The listing builds one solid part. Answer for the finished solid, in the listing's coordinates (mm). A direction names the side the tool comes from. Coordinates: 2 decimals unless noted, no trailing zeros. Loops run counter-clockwise (first coordinate to the right, second up) from the corner with the lowest first, then second, coordinate; pieces in that order, holes last. Notation, with made-up numbers: M 27.5,43.5 L 52.5,43.5 A33 ccw 52.5,78.5 Z; hole C 3.5,19 d9. An arc over 180 degrees is marked long. Return JSON: item names as keys, results as strings. Group by question number.
1. Given P1, Ø1.9, axis at x = -28.375, z = -12, coming from the -Y side; P2, Ø3.5, axis at x = 0, z = 11, coming from the -Y side (3 decimals); P3, Ø6.5, axis at x = 0, z = 19, coming from the +Y side, each flat-ended and moving along its own axis, determine where each tip first touches the part or whether it passes through.
2. Which of the six approach directions +Z, -Z, +X, -X, +Y, -Y give full straight-line access (tool end or side, diameter ignored) to faces 5 (the face through (-2.72, 5.118, 15.453)), 6 (the face through (12.69, 1.61, -12.59)), 7 (the face through (9.487, 4.74, -0.336))?
3. Section D-D (y = 2) is taken. Count the separate pieces of the cut face and the enclosed holes in it, then the cut area to 3 significant figures.
4. The mould has two halves that part along X. Classify faces 1 (the face through (-15.35, 3.13, 20.23)), 2 (the face through (-40, 3, 0)), 3 (the face through (18, 3.85, 2)), 4 (the face through (8, 6.35, -6)): pulls with the +X half, pulls with the -X half, needs draft (parallel to the pull), parting line crosses it, or undercut.
5. Section B-B (z = 20) is taken. Write down the section's boundary in (x, y) (3 decimals).
6. Straight lines are drawn through the part: L1, parallel to X at y = 2.25, z = 20 (3 decimals); L2, parallel to Z at x = -11, y = 5.3; L3, parallel to X at y = 0.75, z = -1.5. For each, find the intervals that lie inside material, in ascending order. Write a range as from..to.
7. Section C-C (z = -3) is taken. Write down the section's boundary in (x, y) (3 decimals).
8. Section A-A (x = 19) is taken. Write down the section's boundary in (y, z).
```python
from build123d import *

# Parameters (mm, degrees)
SKETCH1_W           = 80
SKETCH1_H           = 55
SKETCH1_R           = 1.55
SKETCH1_R_2         = 2.05
SKETCH1_R_3         = 1.05
SKETCH1_R_4         = 1.35
SKETCH1_R_5         = 9
BOSS_EXTRUDE1_DEPTH = 6.35
SKETCH3_R           = 4.47
CUT_EXTRUDE2_DEPTH  = 2.5
SKETCH2_W           = 29
SKETCH2_H           = 29
CUT_EXTRUDE1_DEPTH  = 3.175
FILLET1_R           = 6.35


with BuildPart() as part:
    # Sketch1 → Boss-Extrude1 (new body)
    with BuildSketch(Plane(origin=(0, 0, 0), x_dir=(1, 0, 0), z_dir=(0, 1, 0))):
        Rectangle(SKETCH1_W, SKETCH1_H)
        with Locations(Location((0, 11, 0), (0, 0, 270))):
            Circle(SKETCH1_R, mode=Mode.SUBTRACT)
        with Locations(Location((11, 0, 0), (0, 0, 270))):
            Circle(SKETCH1_R, mode=Mode.SUBTRACT)
        with Locations(Location((0, -11, 0), (0, 0, 270))):
            Circle(SKETCH1_R, mode=Mode.SUBTRACT)
        with Locations(Location((-11, 0, 0), (0, 0, 270))):
            Circle(SKETCH1_R, mode=Mode.SUBTRACT)
        with Locations(Location((0, 19, 0), (0, 0, 270))):
            Circle(SKETCH1_R_2, mode=Mode.SUBTRACT)
        with Locations(Location((19, 0, 0), (0, 0, 270))):
            Circle(SKETCH1_R_2, mode=Mode.SUBTRACT)
        with Locations(Location((0, -19, 0), (0, 0, 270))):
            Circle(SKETCH1_R_2, mode=Mode.SUBTRACT)
        with Locations(Location((-19, 0, 0), (0, 0, 270))):
            Circle(SKETCH1_R_2, mode=Mode.SUBTRACT)
        with Locations(Location((37.017505191, 23.98740934, 0), (0, 0, 270))):
            Circle(SKETCH1_R_3, mode=Mode.SUBTRACT)
        with Locations(Location((-36.555321603, 23.98740934, 0), (0, 0, 270))):
            Circle(SKETCH1_R_4, mode=Mode.SUBTRACT)
        with Locations(Location((-36.939866092, -23.51259066, 0), (0, 0, 270))):
            Circle(SKETCH1_R_4, mode=Mode.SUBTRACT)
        with Locations(Location((0, 0, 0), (0, 0, 270))):
            Circle(SKETCH1_R_5, mode=Mode.SUBTRACT)
        with Locations(Location((16.375, -20, 0), (0, 0, 270))):
            Circle(SKETCH1_R_3, mode=Mode.SUBTRACT)
        with Locations(Location((28.375, -12, 0), (0, 0, 270))):
            Circle(SKETCH1_R_3, mode=Mode.SUBTRACT)
        with Locations(Location((28.375, -20, 0), (0, 0, 270))):
            Circle(SKETCH1_R_3, mode=Mode.SUBTRACT)
        with Locations(Location((28.375, 20, 0), (0, 0, 90))):
            Circle(SKETCH1_R_3, mode=Mode.SUBTRACT)
        with Locations(Location((28.375, 12, 0), (0, 0, 90))):
            Circle(SKETCH1_R_3, mode=Mode.SUBTRACT)
        with Locations(Location((16.375, 20, 0), (0, 0, 90))):
            Circle(SKETCH1_R_3, mode=Mode.SUBTRACT)
        with Locations(Location((-28.375, -20, 0), (0, 0, 90))):
            Circle(SKETCH1_R_3, mode=Mode.SUBTRACT)
        with Locations(Location((-28.375, -12, 0), (0, 0, 90))):
            Circle(SKETCH1_R_3, mode=Mode.SUBTRACT)
        with Locations(Location((-16.375, -20, 0), (0, 0, 90))):
            Circle(SKETCH1_R_3, mode=Mode.SUBTRACT)
        with Locations(Location((-16.375, 20, 0), (0, 0, 270))):
            Circle(SKETCH1_R_3, mode=Mode.SUBTRACT)
        with Locations(Location((-28.375, 12, 0), (0, 0, 270))):
            Circle(SKETCH1_R_3, mode=Mode.SUBTRACT)
        with Locations(Location((-28.375, 20, 0), (0, 0, 270))):
            Circle(SKETCH1_R_3, mode=Mode.SUBTRACT)
        with Locations(Location((37.017505191, -0.577084193, 0), (0, 0, 270))):
            Circle(SKETCH1_R_3, mode=Mode.SUBTRACT)
    extrude(amount=BOSS_EXTRUDE1_DEPTH)

    # Sketch3 → Cut-Extrude2 (cut)
    with BuildSketch(Plane(origin=(0, 6.35, 0), x_dir=(1, 0, 0), z_dir=(0, 1, 0))):
        with Locations(Location((0, -19, 0), (0, 0, 270))):
            Circle(SKETCH3_R)
        with Locations(Location((19, 0, 0), (0, 0, 270))):
            Circle(SKETCH3_R)
        with Locations(Location((-19, 0, 0), (0, 0, 270))):
            Circle(SKETCH3_R)
        with Locations(Location((0, 19, 0), (0, 0, 270))):
            Circle(SKETCH3_R)
    extrude(amount=-CUT_EXTRUDE2_DEPTH, mode=Mode.SUBTRACT)

    # Sketch2 → Cut-Extrude1 (cut)
    with BuildSketch(Plane.XZ):
        Rectangle(SKETCH2_W, SKETCH2_H)
    extrude(amount=-CUT_EXTRUDE1_DEPTH, mode=Mode.SUBTRACT)

    # Fillet1
    fillet1_edges = [part.edges().sort_by_distance(p)[0] for p in [
        (14.5, 1.5875, 14.5),
        (14.5, 1.5875, -14.5),
        (-14.5, 1.5875, -14.5),
        (-14.5, 1.5875, 14.5),
    ]]
    fillet(fillet1_edges, radius=FILLET1_R)


solid = part.part
```
Worked out:
{
 "1": {"P1": "through", "P2": "y = 3.175", "P3": "y = 3.85"},
 "2": {"face 5": "+Y", "face 6": "-Y", "face 7": "+Y, -Y"},
 "3": {"separate pieces": "1", "enclosed holes": "21", "area": "3,480 mm^2"},
 "4": {"face 1": "undercut", "face 2": "pulls with the -X half", "face 3": "undercut", "face 4": "needs draft"},
 "5": {"outline": "M -40,0 L -29.425,0 L -29.425,6.35 L -40,6.35 Z; M -27.325,0 L -17.425,0 L -17.425,6.35 L -27.325,6.35 Z; M -15.325,0 L -1.79,0 L -1.79,3.85 L -4.357,3.85 L -4.357,6.35 L -15.325,6.35 Z; M 1.79,0 L 15.325,0 L 15.325,6.35 L 4.357,6.35 L 4.357,3.85 L 1.79,3.85 Z; M 17.425,0 L 27.325,0 L 27.325,6.35 L 17.425,6.35 Z; M 29.425,0 L 40,0 L 40,6.35 L 29.425,6.35 Z"},
 "6": {"L1": "-40..-29.425, -27.325..-17.425, -15.325..-1.79, 1.79..15.325, 17.425..27.325, 29.425..40", "L2": "-27.5..-1.55, 1.55..27.5", "L3": "-40..-20.4, -17.6..-14.5, 14.5..17.6, 20.4..40"},
 "7": {"outline": "M -40,0 L -14.5,0 L -14.5,3.175 L -8.485,3.175 L -8.485,6.35 L -15.686,6.35 L -15.686,3.85 L -22.314,3.85 L -22.314,6.35 L -40,6.35 Z; M 8.485,3.175 L 14.5,3.175 L 14.5,0 L 40,0 L 40,6.35 L 22.314,6.35 L 22.314,3.85 L 15.686,3.85 L 15.686,6.35 L 8.485,6.35 Z"},
 "8": {"outline": "M 0,-27.5 L 6.35,-27.5 L 6.35,-4.47 L 3.85,-4.47 L 3.85,-2.05 L 0,-2.05 Z; M 0,2.05 L 3.85,2.05 L 3.85,4.47 L 6.35,4.47 L 6.35,27.5 L 0,27.5 Z"}
}
